```python
from build123d import *

# Parameters (mm, degrees)
SKETCH1_R           = 7.5
BOSS_EXTRUDE1_DEPTH = 9.5
SKETCH2_R           = 1.5875


with BuildPart() as part:
    # Sketch1 → Boss-Extrude1 (new body)
    with BuildSketch(Plane(origin=(0, 0, 0), x_dir=(1, 0, 0), z_dir=(0, 1, 0))):
        Circle(SKETCH1_R)
        with BuildLine():
            Line((-2, 1.5), (2, 1.5))
            ThreePointArc((2, 1.5), (2.5, 0), (2, -1.5))
            Line((2, -1.5), (-2, -1.5))
            ThreePointArc((-2, -1.5), (-2.5, 0), (-2, 1.5))
        make_face(mode=Mode.SUBTRACT)
    extrude(amount=BOSS_EXTRUDE1_DEPTH)

    # Sketch2 → Cut-Revolve1 (revolve, cut)
    with BuildSketch(Plane.XY):
        with Locations((7.5, 4.75)):
            Circle(SKETCH2_R)
    revolve(axis=Axis((0, 9.5, 0), (0, -1, 0)), mode=Mode.SUBTRACT)


solid = part.part
```
Geometry check sheet. Reference: the model listing, model coordinates, mm. A direction names the side the tool comes from. Give positions to 0.01 mm unless a question says otherwise; leave off trailing zeros. Order: outer loops, then holes, each group sorted by start corner. A loop starts at its lowest first (then second) coordinate and runs counter-clockwise, first axis right, second up. Notation, with made-up numbers: (-26.75, 47.5) - (-14.75, 47.5) arc R10 cw to (-14.75, 62.5) - close; hole circle Ø10 at (6.25, -24). An arc over 180 degrees is marked (long way). Write item = value, one per line. Start each with the question number.
1) Access from +Z, -Z, +X, -X, +Y, -Y to the whole of each face (thin tool, end or side, straight path). Record for faces 4 (the flat face through (0, 9.5, 2)), 5 (the cylindrical face through (-2.5, 4.7, 0)).
2) Gauge pin test, flat ends, axial feed: pin 1 Ø1 at (x, y) = (2, 2) entering from +Z; pin 2 Ø5 at (y, z) = (4, -5) entering from +X; pin 3 Ø1 at (x, y) = (-1, 3) entering from +Z. Record the tip position at first contact, or that the pin passes through.
3) Section check C-C (y = 7). Enter the section's corners in (x, z), then the cut area to 3 significant figures.
4) Scan lines: L1, parallel to Z at x = -0.25, y = 7.25; L2, parallel to Y at x = -3, z = 6.75; L3, parallel to Y at x = 5.25, z = 3.75. Record each from-to range of solid material in increasing order.
5) Section check D-D (y = 5.5). Enter the section's corners in (x, z), then the cut area to 3 significant figures.
6) Draft check along Z on faces 1 (the flat face through (0, 0, 2)), 2 (the flat face through (0, 5, 1.5)), 3 (the cylindrical face through (-7.493, 7.897, -0.33)). Enter one of: released by +Z, released by -Z, zero draft, split by the parting line, or undercut.
Geometry check:
q1.face_4 = +Z, -Z, +X, -X, +Y
q1.face_5 = +Y, -Y
q2.pin_1 = 7.35
q2.pin_2 = 7.02
q2.pin_3 = 7.48
q3.outline = circle Ø15 at (0, 0); hole (-2, -1.5) - (2, -1.5) arc R2.5 ccw to (2, 1.5) - (-2, 1.5) arc R2.5 ccw to start
q3.area = 163 mm2
q4.L1 = -7.5 to -1.5, 1.5 to 7.5
q4.L2 = 0 to 3.17, 6.33 to 9.5
q4.L3 = 0 to 3.56, 5.94 to 9.5
q5.outline = circle Ø12.2 at (0, 0); hole (-2, -1.5) - (2, -1.5) arc R2.5 ccw to (2, 1.5) - (-2, 1.5) arc R2.5 ccw to start
q5.area = 103 mm2
q6.face_1 = zero draft
q6.face_2 = undercut
q6.face_3 = split by the parting line
